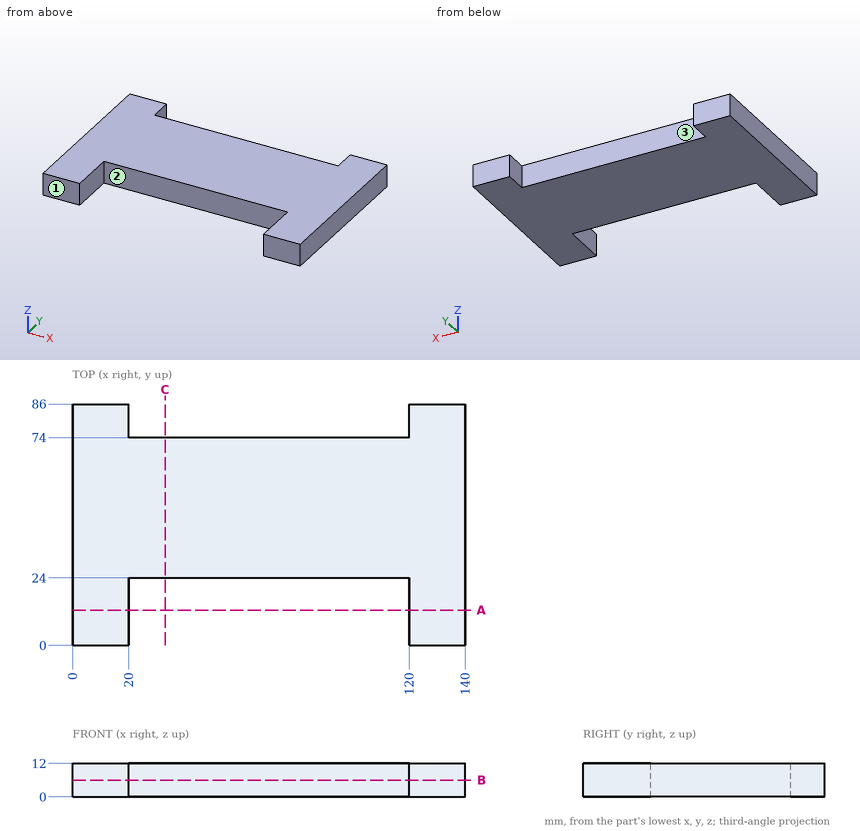
Here's the drawing with two shaded views (mm, measured from the low corner). I have some questions. A direction names the side the tool comes from. Give positions to 0.01 mm unless a question says otherwise; leave off trailing zeros. Order: outer loops, then holes, each group sorted by start corner. A loop starts at its lowest first (then second) coordinate and runs counter-clockwise, first axis right, second up. Notation, with made-up numbers: (-40, 55) -> (10, 55) arc R13 ccw to (10, 69) -> close; hole circle Ø6 at (50.25, 62.5). An arc over 180 degrees is marked (long way). Use a Markdown table: item, result. Add a question column.
Item 1: Imagine slicing it at B-B on z = 6. Please give me the cut outline in (x, y).
Item 2: I need wall thicknesses on line 1 (X direction, y = 77, z = 1); line 2 (Y direction, x = 61.5, z = 8). Which ranges of each line are inside material? Lowest first, please.
Item 3: Imagine slicing it at A-A on y = 12.5. Please give me the cut outline in (x, z).
Item 4: For the marked faces 1, 2 and 3, which set-ups out of +Z, -Z, +X, -X, +Y, -Y let a thin tool reach every point of the face, with its end or its side?
Item 5: Imagine slicing it at C-C on x = 33. Please give me the cut outline in (y, z), plus the area to 3 significant figures.
Item 6: Will these pins go through, and if not, where does the flat tip stop? pin 1 (6 mm diameter, centred on x = 96.5, z = 6, fed in from -Y); pin 2 (1 mm diameter, centred on x = 57, z = 5.5, fed in from +Y).
Data:
| question | item | result |
|---|---|---|
| 1 | outline | (0, 0) -> (20, 0) -> (20, 24) -> (120, 24) -> (120, 0) -> (140, 0) -> (140, 86) -> (120, 86) -> (120, 74) -> (20, 74) -> (20, 86) -> (0, 86) -> close |
| 2 | line 1 | x = 0 to 20, 120 to 140 |
| 2 | line 2 | y = 24 to 74 |
| 3 | outline | (0, 0) -> (20, 0) -> (20, 12) -> (0, 12) -> close; (120, 0) -> (140, 0) -> (140, 12) -> (120, 12) -> close |
| 4 | face 1 | +Z, -Z, +X, -X, -Y |
| 4 | face 2 | +Z, -Z, -Y |
| 4 | face 3 | +Z, -Z, +Y |
| 5 | outline | (24, 0) -> (74, 0) -> (74, 12) -> (24, 12) -> close |
| 5 | area | 600 mm² |
| 6 | pin 1 | stops at y = 24 |
| 6 | pin 2 | stops at y = 74 |
